CAD build for the part. Positions are in the model's coordinates, mm. A direction names the side the tool comes from. Coordinates: 2 decimals unless noted, no trailing zeros. Write each loop counter-clockwise with the first axis right and the second up, starting at its lowest first coordinate (ties: lowest second). Pieces come first, ordered by that corner, then holes. Notation, with made-up numbers: M 45.5,-40 L 72.5,-40 A11 ccw 72.5,-34 Z; hole C -4,3 d2. An arc over 180 degrees is marked long. Put each result on its own line as item: value. Start each with the question number.
```python
from build123d import *

# Parameters (mm, degrees)
F0_W     = 115.57
F0_H     = 56.388
F1_DEPTH = 8.636
F3_DEPTH = 104.14
F5_DEPTH = 7.62
F7_DEPTH = 7.62


with BuildPart() as f1:
    # F0 (on Top) → F1 (new body)
    with BuildSketch(Plane.XY):
        with Locations((-57.785, -28.194)):
            Rectangle(F0_W, F0_H)
    extrude(amount=F1_DEPTH)

    # F2 (on face) → F3 (join)
    with BuildSketch(Plane.XY.offset(8.636)):
        Polygon((0, -56.388), (0, -28.194), (0, 0), (-10.16, 0), (-10.16, -5.08), (-5.08, -5.08), (-5.08, -2.54), (-2.54, -2.54), (-2.54, -28.194), (-2.54, -53.848), (-5.08, -53.848), (-5.08, -51.308), (-10.16, -51.308), (-10.16, -56.388), align=None)
        Polygon((-105.41, -5.08), (-105.41, 0), (-115.57, 0), (-115.57, -28.194), (-115.57, -56.388), (-105.41, -56.388), (-105.41, -51.308), (-110.49, -51.308), (-110.49, -53.848), (-113.03, -53.848), (-113.03, -28.194), (-113.03, -2.54), (-110.49, -2.54), (-110.49, -5.08), align=None)
    extrude(amount=F3_DEPTH)

    # F4 (on face) → F5 (join)
    with BuildSketch(Plane.YZ.offset(-113.03)):
        with BuildLine():
            Line((-53.848, 8.636), (-28.194, 8.636))
            Line((-28.194, 8.636), (-2.54, 8.636))
            Line((-2.54, 8.636), (-25.280232, 24.558882))
            ThreePointArc((-25.280232, 24.558882), (-26.666415, 25.242471), (-28.194, 25.477589))
            ThreePointArc((-28.194, 25.477589), (-29.721585, 25.242471), (-31.107768, 24.558882))
            Line((-31.107768, 24.558882), (-53.848, 8.636))
        make_face()
    extrude(amount=F5_DEPTH)

    # F6 (on face) → F7 (join)
    with BuildSketch(Plane(origin=(-2.54, 0, 0), x_dir=(0, -1, 0), z_dir=(-1, 0, 0))):
        with BuildLine():
            Line((2.54, 8.636), (28.194, 8.636))
            Line((28.194, 8.636), (53.848, 8.636))
            Line((53.848, 8.636), (31.107768, 24.558882))
            ThreePointArc((31.107768, 24.558882), (29.721585, 25.242471), (28.194, 25.477589))
            ThreePointArc((28.194, 25.477589), (26.666415, 25.242471), (25.280232, 24.558882))
            Line((25.280232, 24.558882), (2.54, 8.636))
        make_face()
    extrude(amount=F7_DEPTH)


solid = f1.part
```
(1) Slice it at C-C, the plane x = -12. Write the cut outline in (y, z), then the cut area to 3 significant figures.
(2) Which spindle directions (+Z, -Z, +X, -X, +Y, -Y) get a long thin tool onto all of the face, cutting with end or side? Do faces 1 (the face through (-10.16, -28, 22)), 2 (the face through (0, -29, 56)), 3 (the face through (-113.03, -29, 60)). Say none if no direction does.
(3) Two-plate mould, pull along X, no slides. Class faces 4 (the face through (-115.57, -29, 56)), 5 (the face through (-105.41, -28, 22)), 6 (the face through (-59, -28, 0)): +X half, -X half, draft (parallel to the pull), parting line (faces both ways), or undercut.
(4) Drill centre lines: line 1 (X direction, y = -38, z = 37); line 2 (Y direction, x = -7.5, z = 86); line 3 (X direction, y = -54, z = 47). Where is each one in solid material? Low to high. Write a range as [from, to].
(5) Slice it at A-A, the plane z = 68.5. Write the cut outline in (x, y), then the cut area to 3 significant figures.
(6) Slice it at B-B, the plane y = -40.5. Write the cut outline in (x, z).
(7) Drop a flat-ended pin along its axis: pin 1 (8 mm diameter, centred on x = -66, y = -33, fed in from +Z). Give the stop position or say it passes through.
Result set:
1. outline: M -56.39,0 L 0,0 L 0,8.64 L -56.39,8.64 Z
1. area: 487 mm^2
2. face 1: +Z, +Y, -Y
2. face 2: +Z, -Z, +X, +Y, -Y
2. face 3: +Z
3. face 4: -X half
3. face 5: undercut
3. face 6: draft
4. line 1: x = [-115.57, -113.03], [-2.54, 0]
4. line 2: y = [-56.39, -51.31], [-5.08, 0]
4. line 3: x = [-115.57, -105.41], [-10.16, 0]
5. outline: M -115.57,-56.39 L -105.41,-56.39 L -105.41,-51.31 L -110.49,-51.31 L -110.49,-53.85 L -113.03,-53.85 L -113.03,-2.54 L -110.49,-2.54 L -110.49,-5.08 L -105.41,-5.08 L -105.41,0 L -115.57,0 Z; M -10.16,-56.39 L 0,-56.39 L 0,0 L -10.16,0 L -10.16,-5.08 L -5.08,-5.08 L -5.08,-2.54 L -2.54,-2.54 L -2.54,-53.85 L -5.08,-53.85 L -5.08,-51.31 L -10.16,-51.31 Z
5. area: 415 mm^2
6. outline: M -115.57,0 L 0,0 L 0,112.78 L -2.54,112.78 L -2.54,17.98 L -10.16,17.98 L -10.16,8.64 L -105.41,8.64 L -105.41,17.98 L -113.03,17.98 L -113.03,112.78 L -115.57,112.78 Z
7. pin 1: stops at z = 8.64
